Here's how the part is built. I have some questions about the finished solid (model axes, mm). Face numbers are marked on the shaded views. Give positions to 0.01 mm unless a question says otherwise; leave off trailing zeros. Write each loop counter-clockwise with the first axis right and the second up, starting at its lowest first coordinate (ties: lowest second). Pieces come first, ordered by that corner, then holes. Notation, with made-up numbers: (38, -2) -> (73, -2) arc R20 cw to (73, 28) -> close; hole circle Ø11 at (50.5, 32.25). An arc over 180 degrees is marked (long way). Return JSON: item names as keys, results as strings.
from build123d import *

# Parameters (mm, degrees)
CURVED_PLATE_DEPTH   = 190
IR_CUTOUT_DEPTH      = 20
SKETCH3_R            = 3.5687
MOUNTING_HOLES_DEPTH = 66.75


with BuildPart() as part:
    # Sketch1 → Curved Plate (new body)
    with BuildSketch(Plane(origin=(0, 0, 0), x_dir=(1, 0, 0), z_dir=(0, 1, 0))):
        with BuildLine():
            Line((170.139573777, 0), (175, 0))
            ThreePointArc((175, 0), (0, 65.75), (-175, 0))
            Line((-175, 0), (-170.139573777, 0))
            ThreePointArc((-170.139573777, 0), (0, 62.575), (170.139573777, 0))
        make_face()
    extrude(amount=CURVED_PLATE_DEPTH)

    # Sketch2 → IR Cutout (cut)
    with BuildSketch(Plane(origin=(0, 0, 0), x_dir=(1, 0, 0), z_dir=(0, 1, 0))):
        with BuildLine():
            Line((-117.762328859, 38.234983169), (-105.521942389, 25.994596699))
            Line((-105.521942389, 25.994596699), (-101.986408483, 22.459062793))
            Line((-101.986408483, 22.459062793), (-73.702137236, 50.743334041))
            Line((-73.702137236, 50.743334041), (-77.237671141, 54.278867947))
            ThreePointArc((-77.237671141, 54.278867947), (-97.829451392, 47.089074697), (-117.762328859, 38.234983169))
        make_face()
        with BuildLine():
            Line((77.237671141, 54.278867947), (73.702137236, 50.743334041))
            Line((73.702137236, 50.743334041), (101.986408483, 22.459062793))
            Line((101.986408483, 22.459062793), (105.521942389, 25.994596699))
            Line((105.521942389, 25.994596699), (117.762328859, 38.234983169))
            ThreePointArc((117.762328859, 38.234983169), (97.829451392, 47.089074697), (77.237671141, 54.278867947))
        make_face()
        with BuildLine():
            Line((-20, 64.996386215), (-20, 59.996386215))
            Line((-20, 59.996386215), (20, 59.996386215))
            Line((20, 59.996386215), (20, 64.996386215))
            ThreePointArc((20, 64.996386215), (0, 65.75), (-20, 64.996386215))
        make_face()
    extrude(amount=IR_CUTOUT_DEPTH, mode=Mode.SUBTRACT)

    # Sketch3 → Mounting Holes (cut, through all)
    with BuildSketch(Plane.XY):
        with Locations((-159.125, 164.6)):
            Circle(SKETCH3_R)
        with Locations((-159.125, 25.4)):
            Circle(SKETCH3_R)
        with Locations((159.125, 25.4)):
            Circle(SKETCH3_R)
        with Locations((159.125, 164.6)):
            Circle(SKETCH3_R)
    extrude(amount=-MOUNTING_HOLES_DEPTH, mode=Mode.SUBTRACT)


solid = part.part
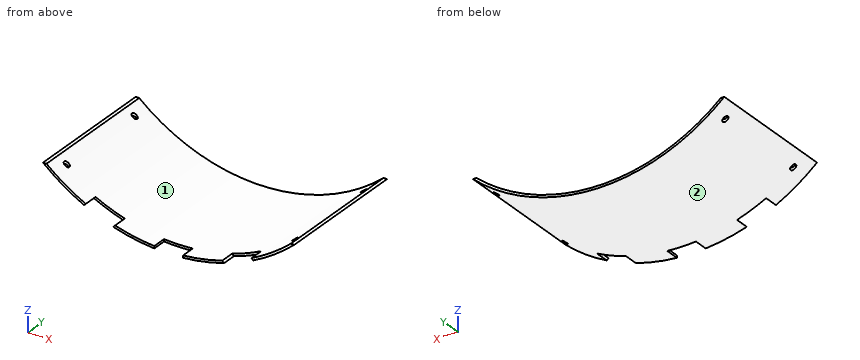
1. Suppose I cut it at B-B, the plane y = 25.4. List the corners of the cut face in (x, z) for me.
Taken from the geometry:
{"outline": "(-175, 0) arc R265.76 ccw to (-162.69, -10.13) -> (-162.69, -6.1) arc R262.59 cw to (-170.14, 0) -> close; (-155.56, -15.47) arc R265.76 ccw to (155.56, -15.47) -> (155.56, -11.54) arc R262.59 cw to (-155.56, -11.54) -> close; (162.69, -10.13) arc R265.76 ccw to (175, 0) -> (170.14, 0) arc R262.59 cw to (162.69, -6.1) -> close"}
2. If we mould it in two halves opening along X, with no side actions, what happens to the marked faces 1 and 2? For each: released by +X, released by -X, zero draft, split by the parting line, or undercut.
Taken from the geometry:
{"face 1": "undercut", "face 2": "split by the parting line"}
3. Suppose I cut it at C-C, the plane x = -107. List the corners of the cut face in (y, z) for me, and give its area (3 significant figures).
Taken from the geometry:
{"outline": "(20, -43.26) -> (190, -43.26) -> (190, -39.79) -> (20, -39.79) -> close", "area": "590 mm²"}
4. If I drill on line 1 (X direction, y = 25.4, z = -13.25); line 2 (Z direction, x = 4.5, y = 118.5); line 3 (X direction, y = 58, z = -31.5), over which ranges is the centre line in solid material (lowest first)? Write a range as [from, to].
Taken from the geometry:
{"line 1": "x = [-155.56, -153.2], [153.2, 155.56]", "line 2": "z = [-65.71, -62.54]", "line 3": "x = [-130.51, -123.91], [123.91, 130.51]"}
5. Suppose I cut it at A-A, the plane z = -19. List the corners of the cut face in (x, y) for me.
Taken from the geometry:
{"outline": "(-150.54, 0) -> (-144.87, 0) -> (-144.87, 190) -> (-150.54, 190) -> close; (144.87, 0) -> (150.54, 0) -> (150.54, 190) -> (144.87, 190) -> close"}
6. For pin 1 Ø6 at (x, y) = (-32, 139) entering from +Z; pin 2 Ø2 at (y, z) = (39.5, -22.5) entering from +X; pin 3 Ø8 at (x, y) = (159.125, 25.4) entering from +Z, each with a flat end and sliding along its axis, tell me the tip position at first contact or that it passes through.
Taken from the geometry:
{"pin 1": "stops at z = -60.23", "pin 2": "stops at x = 146.84", "pin 3": "stops at z = -5.76"}
7. Suppose I cut it at D-D, the plane x = 35. List the corners of the cut face in (y, z) for me.
Taken from the geometry:
{"outline": "(0, -63.44) -> (190, -63.44) -> (190, -60.23) -> (0, -60.23) -> close"}
